Read the model definition and answer for the solid it produces. Units are mm, in the model's axes. A direction names the side the tool comes from. Coordinates: 2 decimals unless noted, no trailing zeros. Loops run counter-clockwise (first coordinate to the right, second up) from the corner with the lowest first, then second, coordinate; pieces in that order, holes last.
from build123d import *

# Parameters (mm, degrees)
EXTRUDE_1_DEPTH     = 4.5
FILLET_1_R          = 20
SKETCH_2_W          = 10
SKETCH_2_H          = 10
CUT_EXTRUDE_1_DEPTH = 116.19657113
SKETCH_3_R          = 1.75
CUT_EXTRUDE_2_DEPTH = 116.19657113


with BuildPart() as part:
    # 스케치1 → 보스-돌출1 (new body)
    with BuildSketch(Plane(origin=(0, 0, 0), x_dir=(1, 0, 0), z_dir=(0, 1, 0))):
        with BuildLine():
            Line((-65, 25), (-34.194351712, 75.754428709))
            ThreePointArc((-34.194351712, 75.754428709), (0, 95), (34.194351712, 75.754428709))
            Line((34.194351712, 75.754428709), (65, 25))
            Line((65, 25), (65, -75))
            Line((65, -75), (-65, -75))
            Line((-65, -75), (-65, 25))
        make_face()
    extrude(amount=EXTRUDE_1_DEPTH)

    # 필렛1
    fillet_1_edges = [part.edges().sort_by_distance(p)[0] for p in [
        (-65, 2.25, -25),
        (65, 2.25, -25),
    ]]
    fillet(fillet_1_edges, radius=FILLET_1_R)

    # 스케치2 → 컷-돌출1 (cut, through all)
    with BuildSketch(Plane(origin=(0, 4.5, 0), x_dir=(1, 0, 0), z_dir=(0, 1, 0))):
        with Locations((-60, 11.5)):
            Rectangle(SKETCH_2_W, SKETCH_2_H)
        with Locations((60, 11.5)):
            Rectangle(SKETCH_2_W, SKETCH_2_H)
    extrude(amount=-CUT_EXTRUDE_1_DEPTH, mode=Mode.SUBTRACT)

    # 스케치3 → 컷-돌출2 (cut, through all)
    with BuildSketch(Plane(origin=(0, 4.5, 0), x_dir=(1, 0, 0), z_dir=(0, 1, 0))):
        with Locations(Location((-60, -60, 0), (0, 0, 270))):
            Circle(SKETCH_3_R)
        with Locations(Location((-60, -70, 0), (0, 0, 270))):
            Circle(SKETCH_3_R)
        with Locations(Location((60, -60, 0), (0, 0, 270))):
            Circle(SKETCH_3_R)
        with Locations(Location((60, -70, 0), (0, 0, 270))):
            Circle(SKETCH_3_R)
        with Locations(Location((-10, -60, 0), (0, 0, 270))):
            Circle(SKETCH_3_R)
        with Locations(Location((10, -60, 0), (0, 0, 270))):
            Circle(SKETCH_3_R)
        with Locations(Location((-10, -70, 0), (0, 0, 270))):
            Circle(SKETCH_3_R)
        with Locations(Location((10, -70, 0), (0, 0, 270))):
            Circle(SKETCH_3_R)
        with Locations(Location((-45, 15, 0), (0, 0, 270))):
            Circle(SKETCH_3_R)
        with Locations(Location((45, 15, 0), (0, 0, 270))):
            Circle(SKETCH_3_R)
        with Locations(Location((-45, -35, 0), (0, 0, 270))):
            Circle(SKETCH_3_R)
        with Locations(Location((45, -35, 0), (0, 0, 270))):
            Circle(SKETCH_3_R)
    extrude(amount=-CUT_EXTRUDE_2_DEPTH, mode=Mode.SUBTRACT)


solid = part.part
Q1. A cutting plane is placed at C-C (x = 10). Give the vertices of the cut face in (y, z), then the cut area to 3 significant figures.
Findings below:
outline: (0, -93.73) - (4.5, -93.73) - (4.5, 58.25) - (0, 58.25) - close; (0, 61.75) - (4.5, 61.75) - (4.5, 68.25) - (0, 68.25) - close; (0, 71.75) - (4.5, 71.75) - (4.5, 75) - (0, 75) - close
area: 728 mm2
Q2. A cutting plane is placed at B-B (z = 35). Give the vertices of the cut face in (x, y).
Findings below:
outline: (-65, 0) - (-46.75, 0) - (-46.75, 4.5) - (-65, 4.5) - close; (-43.25, 0) - (43.25, 0) - (43.25, 4.5) - (-43.25, 4.5) - close; (46.75, 0) - (65, 0) - (65, 4.5) - (46.75, 4.5) - close
Q3. A cutting plane is placed at D-D (z = 60). Give the vertices of the cut face in (x, y).
Findings below:
outline: (-65, 0) - (-61.75, 0) - (-61.75, 4.5) - (-65, 4.5) - close; (-58.25, 0) - (-11.75, 0) - (-11.75, 4.5) - (-58.25, 4.5) - close; (-8.25, 0) - (8.25, 0) - (8.25, 4.5) - (-8.25, 4.5) - close; (11.75, 0) - (58.25, 0) - (58.25, 4.5) - (11.75, 4.5) - close; (61.75, 0) - (65, 0) - (65, 4.5) - (61.75, 4.5) - close
Q4. Straight lines are drawn through the part: probe 1 along X at (y, z) = (2.75, 35); probe 2 along X at (y, z) = (1.8, 60); probe 3 along Z at (x, y) = (-9.5, 2.1). For each, find the intervals that lie inside material, in ascending order.
Findings below:
probe 1: x = -65 to -46.75, -43.25 to 43.25, 46.75 to 65
probe 2: x = -65 to -61.75, -58.25 to -11.75, -8.25 to 8.25, 11.75 to 58.25, 61.75 to 65
probe 3: z = -93.86 to 58.32, 61.68 to 68.32, 71.68 to 75
Q5. Determine the mould class of faces 4 (the face through (-60, 2, -6.5)), 5 (the face through (64.24, 2.28, -24.87)), 6 (the face through (65, 2, 34)) for opening direction Z: +Z half, -Z half, draft (parallel to the pull), parting line (faces both ways), or undercut.
Findings below:
face 4: undercut
face 5: -Z half
face 6: draft
Q6. A cutting plane is placed at A-A (y = 0.85). Count the separate pieces of the cut face and the enclosed holes in it, then the cut area to 3 significant figures.
Findings below:
separate pieces: 1
enclosed holes: 12
area: 18,600 mm2
Q7. Which of the six approach directions +Z, -Z, +X, -X, +Y, -Y give full straight-line access (tool end or side, diameter ignored) to faces 1 (the face through (55, 2, -11)), 2 (the face through (10.526, 2.282, 61.669)), 3 (the face through (-55, 2, -11))?
Findings below:
face 1: +X, +Y, -Y
face 2: +Y, -Y
face 3: -X, +Y, -Y
Q8. Flat-ended cylindrical pins translate along their axes: pin 1 Ø1 at (y, z) = (3.5, -44.5) entering from +X; pin 2 Ø1.3 at (y, z) = (2, -13) entering from -X. Find the tip coordinate at first contact, or state that the pin passes through.
Findings below:
pin 1: stops at x = 53.47
pin 2: stops at x = -55
